CAD build for the part. Positions are in the model's coordinates, mm. Give positions to 0.01 mm unless a question says otherwise; leave off trailing zeros. Loops run counter-clockwise (first coordinate to the right, second up) from the corner with the lowest first, then second, coordinate; pieces in that order, holes last. Notation, with made-up numbers: (34.25, -28) - (79.25, -28) arc R28 ccw to (79.25, -5) - close; hole circle Ø4 at (51, 37). An arc over 180 degrees is marked (long way). Return JSON: item names as keys, results as strings.
from build123d import *

# Parameters (mm, degrees)
SKETCH2_W               = 381
SKETCH2_H               = 1727.2
BOSS_EXTRUDE1_DEPTH     = 18.288
SKETCH3_W               = 18.288
SKETCH3_H               = 76.2
BOSS_EXTRUDE2_DEPTH     = 18.288
LPATTERN1_COUNT         = 5
LPATTERN1_PITCH         = 381
MIRROR1_COPY_1_SKETCH_W = 18.288
MIRROR1_COPY_1_SKETCH_H = 76.2
MIRROR1_COPY_1_DEPTH    = 18.288
MIRROR1_COPY_2_SKETCH_W = 18.288
MIRROR1_COPY_2_SKETCH_H = 76.2
MIRROR1_COPY_2_DEPTH    = 18.288
MIRROR1_COPY_3_SKETCH_W = 18.288
MIRROR1_COPY_3_SKETCH_H = 76.2
MIRROR1_COPY_3_DEPTH    = 18.288
MIRROR1_COPY_4_SKETCH_W = 18.288
MIRROR1_COPY_4_SKETCH_H = 76.2
MIRROR1_COPY_4_DEPTH    = 18.288
CUT_EXTRUDE2_DEPTH      = 1896.363726014
CUT_EXTRUDE4_DEPTH      = 6.35
SKETCH6_W               = 203.2
SKETCH6_H               = 254
CUT_EXTRUDE5_DEPTH      = 1896.363726014
SKETCH7_R               = 3.175
CUT_EXTRUDE6_DEPTH      = 25.4
FILLET1_R               = 50.8
SKETCH10_W              = 228.6
SKETCH10_H              = 76.2
CUT_EXTRUDE7_DEPTH      = 25.4
FILLET2_R               = 25.4
SKETCH12_R              = 3.175
CUT_EXTRUDE10_DEPTH     = 1896.363726014
SKETCH13_R              = 3.175
CUT_EXTRUDE11_DEPTH     = 1896.363726014


with BuildPart() as part:
    # Sketch2 → Boss-Extrude1 (new body)
    with BuildSketch(Plane.XY):
        with Locations((190.5, 863.6)):
            Rectangle(SKETCH2_W, SKETCH2_H)
    boss_extrude1 = extrude(amount=-BOSS_EXTRUDE1_DEPTH)

    # Sketch3 → Boss-Extrude2 (add)
    with BuildSketch(Plane.XY):
        with Locations((-9.144, 88.9)):
            Rectangle(SKETCH3_W, SKETCH3_H)
    boss_extrude2 = extrude(amount=-BOSS_EXTRUDE2_DEPTH)

    # LPattern1: Boss-Extrude2 ×5
    with Locations(*[(0, i * LPATTERN1_PITCH, 0) for i in range(1, LPATTERN1_COUNT)]):
        add(boss_extrude2)

    # Mirror1: Boss-Extrude1, Boss-Extrude2 across plane
    add(boss_extrude1.mirror(Plane(origin=(381, 0, -18.288), x_dir=(0, 0, 1), z_dir=(1, 0, 0))))
    add(boss_extrude2.mirror(Plane(origin=(381, 0, -18.288), x_dir=(0, 0, 1), z_dir=(1, 0, 0))))

    # Mirror1 copy 1 sketch → Mirror1 copy 1 (add)
    with BuildSketch(Plane(origin=(762, 381, 0), x_dir=(-1, 0, 0), z_dir=(0, 0, 1))):
        with Locations((-9.144, -88.9)):
            Rectangle(MIRROR1_COPY_1_SKETCH_W, MIRROR1_COPY_1_SKETCH_H)
    extrude(amount=-MIRROR1_COPY_1_DEPTH)

    # Mirror1 copy 2 sketch → Mirror1 copy 2 (add)
    with BuildSketch(Plane(origin=(762, 762, 0), x_dir=(-1, 0, 0), z_dir=(0, 0, 1))):
        with Locations((-9.144, -88.9)):
            Rectangle(MIRROR1_COPY_2_SKETCH_W, MIRROR1_COPY_2_SKETCH_H)
    extrude(amount=-MIRROR1_COPY_2_DEPTH)

    # Mirror1 copy 3 sketch → Mirror1 copy 3 (add)
    with BuildSketch(Plane(origin=(762, 1143, 0), x_dir=(-1, 0, 0), z_dir=(0, 0, 1))):
        with Locations((-9.144, -88.9)):
            Rectangle(MIRROR1_COPY_3_SKETCH_W, MIRROR1_COPY_3_SKETCH_H)
    extrude(amount=-MIRROR1_COPY_3_DEPTH)

    # Mirror1 copy 4 sketch → Mirror1 copy 4 (add)
    with BuildSketch(Plane(origin=(762, 1524, 0), x_dir=(-1, 0, 0), z_dir=(0, 0, 1))):
        with Locations((-9.144, -88.9)):
            Rectangle(MIRROR1_COPY_4_SKETCH_W, MIRROR1_COPY_4_SKETCH_H)
    extrude(amount=-MIRROR1_COPY_4_DEPTH)

    # Sketch4 → Cut-Extrude2 (cut, through all)
    with BuildSketch(Plane.XY):
        with BuildLine():
            Line((152.4, 1524), (609.6, 1524))
            ThreePointArc((609.6, 1524), (645.521024484, 1509.121024484), (660.4, 1473.2))
            Line((660.4, 1473.2), (660.4, 1016))
            ThreePointArc((660.4, 1016), (645.521024484, 980.078975516), (609.6, 965.2))
            Line((609.6, 965.2), (152.4, 965.2))
            ThreePointArc((152.4, 965.2), (116.478975516, 980.078975516), (101.6, 1016))
            Line((101.6, 1016), (101.6, 1473.2))
            ThreePointArc((101.6, 1473.2), (116.478975516, 1509.121024484), (152.4, 1524))
        make_face()
    extrude(amount=-CUT_EXTRUDE2_DEPTH, mode=Mode.SUBTRACT)

    # Sketch5 → Cut-Extrude4 (cut)
    with BuildSketch(Plane.XY):
        with BuildLine():
            Line((152.4, 1549.4), (609.6, 1549.4))
            ThreePointArc((609.6, 1549.4), (663.481536726, 1527.081536726), (685.8, 1473.2))
            Line((685.8, 1473.2), (685.8, 1016))
            ThreePointArc((685.8, 1016), (663.481536726, 962.118463274), (609.6, 939.8))
            Line((609.6, 939.8), (152.4, 939.8))
            ThreePointArc((152.4, 939.8), (98.518463274, 962.118463274), (76.2, 1016))
            Line((76.2, 1016), (76.2, 1473.2))
            ThreePointArc((76.2, 1473.2), (98.518463274, 1527.081536726), (152.4, 1549.4))
        make_face()
        with BuildLine():
            Line((152.4, 1524), (609.6, 1524))
            ThreePointArc((609.6, 1524), (645.521024484, 1509.121024484), (660.4, 1473.2))
            Line((660.4, 1473.2), (660.4, 1016))
            ThreePointArc((660.4, 1016), (645.521024484, 980.078975516), (609.6, 965.2))
            Line((609.6, 965.2), (152.4, 965.2))
            ThreePointArc((152.4, 965.2), (116.478975516, 980.078975516), (101.6, 1016))
            Line((101.6, 1016), (101.6, 1473.2))
            ThreePointArc((101.6, 1473.2), (116.478975516, 1509.121024484), (152.4, 1524))
        make_face(mode=Mode.SUBTRACT)
    extrude(amount=-CUT_EXTRUDE4_DEPTH, mode=Mode.SUBTRACT)

    # Sketch6 → Cut-Extrude5 (cut, through all)
    with BuildSketch(Plane.XY):
        with Locations((165.1, 457.2)):
            Rectangle(SKETCH6_W, SKETCH6_H)
    extrude(amount=-CUT_EXTRUDE5_DEPTH, mode=Mode.SUBTRACT)

    # Sketch7 → Cut-Extrude6 (cut)
    with BuildSketch(Plane.XY.offset(-6.35)):
        with Locations((381, 952.5)):
            Circle(SKETCH7_R)
        with Locations((482.6, 952.5)):
            Circle(SKETCH7_R)
        with Locations((584.2, 952.5)):
            Circle(SKETCH7_R)
        with Locations(Location((177.8, 952.5, 0), (0, 0, 180))):
            Circle(SKETCH7_R)
        with Locations(Location((279.4, 952.5, 0), (0, 0, 180))):
            Circle(SKETCH7_R)
        with Locations(Location((584.2, 1536.7, 0), (0, 0, 180))):
            Circle(SKETCH7_R)
        with Locations(Location((482.6, 1536.7, 0), (0, 0, 180))):
            Circle(SKETCH7_R)
        with Locations(Location((381, 1536.7, 0), (0, 0, 180))):
            Circle(SKETCH7_R)
        with Locations((279.4, 1536.7)):
            Circle(SKETCH7_R)
        with Locations((177.8, 1536.7)):
            Circle(SKETCH7_R)
        with Locations((673.1, 1244.832930671)):
            Circle(SKETCH7_R)
        with Locations((673.1, 1359.132930671)):
            Circle(SKETCH7_R)
        with Locations((673.1, 1473.432930671)):
            Circle(SKETCH7_R)
        with Locations((673.1, 1130.532930671)):
            Circle(SKETCH7_R)
        with Locations((673.1, 1016.232930671)):
            Circle(SKETCH7_R)
        with Locations(Location((88.9, 1016.232930671, 0), (0, 0, 180))):
            Circle(SKETCH7_R)
        with Locations(Location((88.9, 1130.532930671, 0), (0, 0, 180))):
            Circle(SKETCH7_R)
        with Locations(Location((88.9, 1244.832930671, 0), (0, 0, 180))):
            Circle(SKETCH7_R)
        with Locations(Location((88.9, 1359.132930671, 0), (0, 0, 180))):
            Circle(SKETCH7_R)
        with Locations(Location((88.9, 1473.432930671, 0), (0, 0, 180))):
            Circle(SKETCH7_R)
        with BuildLine():
            Line((152.4, 965.2), (609.6, 965.2))
            ThreePointArc((609.6, 965.2), (645.521024484, 980.078975516), (660.4, 1016))
            Line((660.4, 1016), (660.4, 1473.2))
            ThreePointArc((660.4, 1473.2), (645.521024484, 1509.121024484), (609.6, 1524))
            Line((609.6, 1524), (152.4, 1524))
            ThreePointArc((152.4, 1524), (116.478975516, 1509.121024484), (101.6, 1473.2))
            Line((101.6, 1473.2), (101.6, 1016))
            ThreePointArc((101.6, 1016), (116.478975516, 980.078975516), (152.4, 965.2))
        make_face()
    extrude(amount=-CUT_EXTRUDE6_DEPTH, mode=Mode.SUBTRACT)

    # Fillet1
    fillet1_edges = [part.edges().sort_by_distance(p)[0] for p in [
        (63.5, 330.2, -9.144),
        (63.5, 584.2, -9.144),
        (266.7, 584.2, -9.144),
        (266.7, 330.2, -9.144),
    ]]
    fillet(fillet1_edges, radius=FILLET1_R)

    # Sketch10 → Cut-Extrude7 (cut)
    with BuildSketch(Plane.XY):
        with Locations((520.7, 749.3)):
            Rectangle(SKETCH10_W, SKETCH10_H)
    extrude(amount=-CUT_EXTRUDE7_DEPTH, mode=Mode.SUBTRACT)

    # Fillet2
    fillet2_edges = [part.edges().sort_by_distance(p)[0] for p in [
        (406.4, 711.2, -9.144),
        (406.4, 787.4, -9.144),
        (635, 787.4, -9.144),
        (635, 711.2, -9.144),
    ]]
    fillet(fillet2_edges, radius=FILLET2_R)

    # Sketch12 → Cut-Extrude10 (cut, through all)
    with BuildSketch(Plane(origin=(0, 0, -18.288), x_dir=(-1, 0, 0), z_dir=(0, 0, -1))):
        with Locations((-584.2, 1657.35)):
            Circle(SKETCH12_R)
        with Locations((-482.6, 1657.35)):
            Circle(SKETCH12_R)
        with Locations((-381, 1657.35)):
            Circle(SKETCH12_R)
        with Locations((-279.4, 1657.35)):
            Circle(SKETCH12_R)
        with Locations((-177.8, 1657.35)):
            Circle(SKETCH12_R)
    extrude(amount=-CUT_EXTRUDE10_DEPTH, mode=Mode.SUBTRACT)

    # Sketch13 → Cut-Extrude11 (cut, through all)
    with BuildSketch(Plane(origin=(0, 0, -18.288), x_dir=(-1, 0, 0), z_dir=(0, 0, -1))):
        with Locations((-373.888, 774.7)):
            Circle(SKETCH13_R)
        with Locations((-323.088, 774.7)):
            Circle(SKETCH13_R)
    extrude(amount=-CUT_EXTRUDE11_DEPTH, mode=Mode.SUBTRACT)


solid = part.part
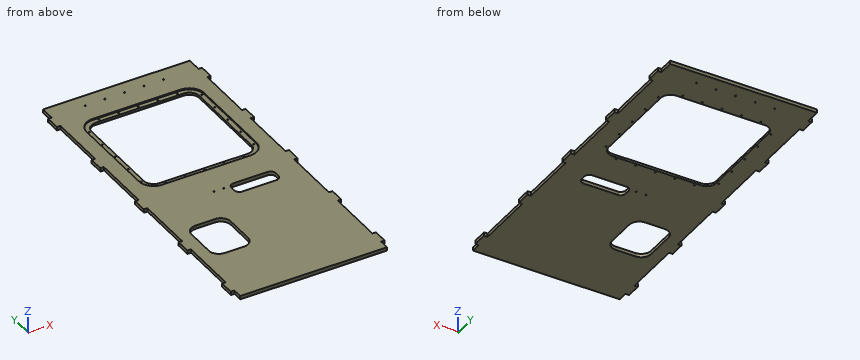
1. Cut at C-C, the plane y = 1507.5. Write the cut outline in (x, z), plus the area to 3 significant figures.
Values follow:
{"outline": "(0, -18.29) - (114.93, -18.29) - (114.93, -6.35) - (84.36, -6.35) - (84.36, 0) - (0, 0) - close; (647.07, -18.29) - (762, -18.29) - (762, 0) - (677.64, 0) - (677.64, -6.35) - (647.07, -6.35) - close", "area": "3,820 mm²"}
2. Cut at A-A, the plane y = 483.5. Write the cut outline in (x, z), plus the area to 3 significant figures.
Values follow:
{"outline": "(-18.29, -18.29) - (63.5, -18.29) - (63.5, 0) - (-18.29, 0) - close; (266.7, -18.29) - (780.29, -18.29) - (780.29, 0) - (266.7, 0) - close", "area": "10,900 mm²"}
3. Cut at D-D, the plane y = 168. Write the cut outline in (x, z), plus the area to 3 significant figures.
Values follow:
{"outline": "(0, -18.29) - (762, -18.29) - (762, 0) - (0, 0) - close", "area": "13,900 mm²"}
4. Drill centre lines: probe 1 along Y at (x, z) = (590, -15.5); probe 2 along X at (y, z) = (952.5, -12.25) (3 decimals); probe 3 along X at (y, z) = (1172.5, -6.75). Where is each one in solid material? Low to high.
Values follow:
{"probe 1": "y = 0 to 711.2, 787.4 to 965.2, 1524 to 1727.2", "probe 2": "x = 0 to 174.625, 180.975 to 276.225, 282.575 to 377.825, 384.175 to 479.425, 485.775 to 581.025, 587.375 to 762", "probe 3": "x = 0 to 101.6, 660.4 to 762"}
5. Drop flat-ended pins along their axis: P1, Ø10, axis at y = 394, z = -4.5, coming from the -X side; P2, Ø4, axis at y = 1480.5, z = -7.5, coming from the +X side; P3, Ø5.5, axis at x = 767, z = -7, coming from the -Y side. Give the stop position or say it passes through.
Values follow:
{"P1": "stops at x = 0", "P2": "stops at x = 762", "P3": "stops at y = 50.8"}
6. Cut at B-B, the plane z = -3.5. Give the number of separate pieces and of enclosed holes in the cut face, plus the area to 3 significant figures.
Values follow:
{"separate pieces": "1", "enclosed holes": "10", "area": "897,000 mm²"}
